Drawing for the job (mm, zero at the part's lowest x, y, z). A direction names the side the tool comes from. Give positions to 0.01 mm unless a question says otherwise; leave off trailing zeros. Order: outer loops, then holes, each group sorted by start corner. A loop starts at its lowest first (then second) coordinate and runs counter-clockwise, first axis right, second up. Notation, with made-up numbers: M 16,84 L 69,84 A36 cw 69,119 Z; hole C -1.75,-13 d1. An arc over 180 degrees is marked long. One line per item, written item: value.
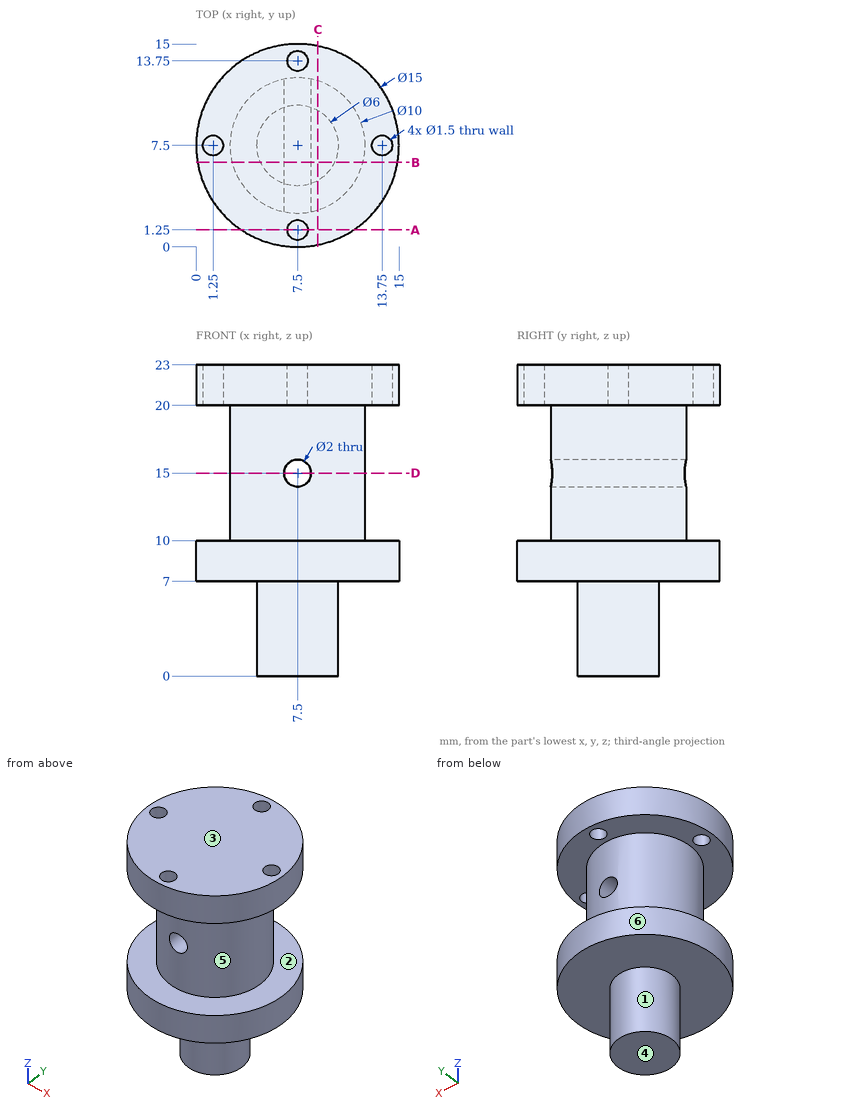
1) Saw through at A-A, the plane y = 1.25. Write the cut outline in (x, z).
Check values:
outline: M 3.35,7 L 11.65,7 L 11.65,10 L 3.35,10 Z; M 3.35,20 L 6.75,20 L 6.75,23 L 3.35,23 Z; M 8.25,20 L 11.65,20 L 11.65,23 L 8.25,23 Z
2) Tool access for the marked faces 1, 2 and 3: list every direction of +Z, -Z, +X, -X, +Y, -Y with a clear straight run to the whole face (end or side of a thin tool).
Check values:
face 1: -Z
face 2: none
face 3: +Z, +X, -X, +Y, -Y
3) Saw through at B-B, the plane y = 6.25. Write the cut outline in (x, z), then the cut area to 3 significant figures.
Check values:
outline: M 0.1,7 L 4.77,7 L 4.77,0 L 10.23,0 L 10.23,7 L 14.9,7 L 14.9,10 L 12.34,10 L 12.34,20 L 14.9,20 L 14.9,23 L 0.1,23 L 0.1,20 L 2.66,20 L 2.66,10 L 0.1,10 Z; hole C 7.5,15 d2
area: 221 mm^2
4) Saw through at D-D, the plane z = 15. Write the cut outline in (x, y), then the cut area to 3 significant figures.
Check values:
outline: M 6.5,2.6 L 6.5,12.4 A5 ccw Z; M 8.5,2.6 A5 ccw 8.5,12.4 Z
area: 58.7 mm^2
5) Mould opens along Z. For the marked faces 4, 5 and 6 say: released by +Z, released by -Z, zero draft, split by the parting line, or undercut.
Check values:
face 4: released by -Z
face 5: undercut
face 6: zero draft
6) Drill centre lines: probe 1 along Z at (x, y) = (4.75, 2); probe 2 along X at (y, z) = (1.25, 21.1); probe 3 along Y at (x, z) = (5.5, 6). Where is each one in solid material? Low to high. Write a range as from..to.
Check values:
probe 1: 7..10, 20..23
probe 2: 3.35..6.75, 8.25..11.65
probe 3: 5.26..9.74
7) Pin check, flat tips, straight feed: pin 1 (2.5 mm diameter, centred on x = 7.5, y = 13.75, fed in from -Z); pin 2 (5 mm diameter, centred on y = 3.5, z = 8, fed in from -X); pin 3 (1.4 mm diameter, centred on x = 13.75, y = 7.5, fed in from +Z); pin 4 (1.2 mm diameter, centred on x = 7.5, z = 15, fed in from +Y). Stop position of each tip, or through.
Check values:
pin 1: z = 7
pin 2: x = 0.15
pin 3: z = 10
pin 4: through
8) Saw through at C-C, the plane x = 9. Write the cut outline in (y, z).
Check values:
outline: M 0.15,7 L 4.9,7 L 4.9,0 L 10.1,0 L 10.1,7 L 14.85,7 L 14.85,10 L 12.27,10 L 12.27,20 L 14.85,20 L 14.85,23 L 0.15,23 L 0.15,20 L 2.73,20 L 2.73,10 L 0.15,10 Z
